Autodesk Inventor part; units mm, degrees
ref_plane "YZ Plane" through (0, 0, 0) normal (1, 0, 0) x (0, 1, 0)
ref_plane "XZ Plane" through (0, 0, 0) normal (0, 1, 0) x (-1, 0, 0)
ref_plane "XY Plane" through (0, 0, 0) normal (0, 0, 1) x (1, 0, 0)
sketch "Base" plane through (0, 0, 0) normal (0, 0, 1) x (1, 0, 0)
  circle A0 centre (0, 0) radius 25.4
  arc A1 (296.4611, -175.8738) -> (140.4514, -91.7589) centre (131.6761, -294.7694) ccw
  arc A2 (110.2711, -36.5273) -> (55.3611, 0.3584) centre (-26.1088, -180.2356) ccw
  arc A3 (110.2711, -36.5273) -> (151.7939, -57.2356) centre (164.9104, 21.0482) ccw
  arc A4 (244.1, -98.1325) -> (151.7939, -57.2356) centre (118.2154, -257.642) ccw
  arc A5 (244.1, -98.1325) -> (322.9398, -136.302) centre (369.9847, 61.3771) ccw
  arc A6 (339.7063, -172.5127) -> (322.9398, -136.302) centre (317.0592, -161.0119) ccw
  arc A7 (296.4611, -175.8738) -> (339.7063, -172.5127) centre (317.0592, -161.0119) ccw
  line L0 (128.6011, -96.3262) -> (140.4514, -91.7589)
  line L1 (0, 0) -> (317.0592, -161.0119) construction
  circle A8 centre (317.0592, -161.0119) radius 25.4 construction
  arc A9 (0, -25.4) -> (128.6011, -96.3262) centre (153.166, 100.265) ccw
  line L2 (0, 0) -> (0, -25.4) construction
  arc A10 (55.3611, 0.3584) -> (42.3326, -1.2004) centre (50.1387, -11.2181) ccw
  arc A11 (25.4, -0.0141) -> (42.3326, -1.2004) centre (34.5266, 8.8174) ccw
  line L3 (110.2711, -36.5273) -> (102.4101, -52.0068) construction
  line L4 (50.1387, -11.2181) -> (44.3883, -22.5417) construction
  line L5 (140.4514, -91.7589) -> (148.7008, -75.5146) construction
  line L6 (244.1, -98.1325) -> (233.6726, -118.6658) construction
  line L7 (339.7063, -172.5127) -> (317.0592, -161.0119) construction
  dimension "d101" = 50.8
  dimension "d98" = 355.6
  dimension "d99" = 203.2
  dimension "d100" = 79.375
  dimension "d102" = 198.12
  dimension "d103" = 50.8
  dimension "d104" = 12.7
  dimension "d105" = 203.2
  dimension "d106" = 48
  dimension "d107" = 12.7
  dimension "d108" = 12.7
  dimension "d109" = 23.495
  dimension "d111" = 158.75
  dimension "d112" = 222.25
  dimension "d113" = 49.784
  dimension "d114" = 65.0748
  dimension "d115" = 51.9176
  dimension "d116" = 95.3008
  dimension "d117" = 93.5228
extrude "Plate1" add sketch "Base" along normal blind 5
sketch "MountHoles" plane through (0, 0, 5) normal (0, 0, 1) x (1, 0, 0)
  arc A0 (296.4611, -175.8738) -> (322.9398, -136.302) centre (317.0592, -161.0119) ccw
  circle A1 centre (317.0592, -161.0119) radius 3.175
  circle A2 centre (0, 0) radius 3.175
  circle A3 centre (0, 0) radius 15.875 construction
  circle A4 centre (0, 15.875) radius 3.175
  line L0 (0, 15.875) -> (0, 0) construction
  circle A5 centre (-13.7482, 7.9375) radius 3.175
  circle A6 centre (-13.7482, -7.9375) radius 3.175
  circle A7 centre (0, -15.875) radius 3.175
  circle A8 centre (13.7482, -7.9375) radius 3.175
  circle A9 centre (13.7482, 7.9375) radius 3.175
  point P0 (278.6053, -195.7416)
  point P1 (14.9365, 6.9557)
  dimension "d40" = 31.75
  dimension "d38" = 6.35
  dimension "d39" = 6.35
  dimension "d43" = 360
hole "MountHolesFeature" at (0, 0, 5) direction (0, 0, -1) diameter 8 end through all
fillet "SmallFilletsFeature" radius 8 2 edges at (140.4514, -91.7589, 2.5) (128.6011, -96.3262, 2.5)
sketch "WheelMountHole" plane through (0, 0, 5) normal (0, 0, 1) x (1, 0, 0)
  arc A0 (296.4611, -175.8738) -> (322.9398, -136.302) centre (317.0592, -161.0119) ccw
  circle A1 centre (317.0592, -161.0119) radius 6.35
  point P0 (0, 0)
  point P1 (278.6053, -195.7416)
  dimension "d83" = 12.7
hole "WheelMountHoleFeature" at (317.0592, -161.0119, 5) direction (0, 0, -1) diameter 24.5 end through all
sketch "PistonMountHole" plane through (0, 0, 0) normal (0, 0, -1) x (-1, 0, 0)
  circle A0 centre (-195.6083, -86.6143) radius 3
  arc A1 (-151.7939, -57.2356) -> (-244.1, -98.1325) centre (-118.2154, -257.642) ccw
  line L0 (-206.4619, -74.6043) -> (-184.7548, -98.6243) construction
  arc A2 (-142.169, -91.8405) -> (-296.4611, -175.8738) centre (-131.6761, -294.7694) ccw
  point P0 (0, 0)
  dimension "d120" = 6
  dimension "d122" = 203.2
  dimension "d197" = 77.3929
extrude "PistonMountHoleFeature" cut sketch "PistonMountHole" against normal blind 5
sketch "MotorExtend" plane through (0, 0, 5) normal (0, 0, 1) x (1, 0, 0)
  circle A0 centre (70.2482, -45.9648) radius 36
  arc A1 (0, -25.4) -> (126.5447, -96.0583) centre (153.166, 100.265) ccw construction
  arc A2 (110.2711, -36.5273) -> (151.7939, -57.2356) centre (164.9104, 21.0482) ccw construction
  circle A3 centre (0, 0) radius 4
  line L0 (0, 0) -> (140.4963, -91.9296) construction
  arc A4 (142.169, -91.8405) -> (138.8789, -92.365) centre (141.7559, -99.8298) ccw
  arc A5 (0, -25.4) -> (46.966, -73.4228) centre (280.2614, 201.7164) ccw
  arc A6 (126.5447, -96.0583) -> (130.4966, -95.5956) centre (127.6196, -88.1308) ccw
  arc A7 (58.6335, -80.0397) -> (126.5447, -96.0583) centre (175.0163, 261.4034) ccw
  arc A8 (55.3611, 0.3584) -> (42.3326, -1.2004) centre (50.1387, -11.2181) ccw
  arc A9 (85.2601, -13.2441) -> (55.3611, 0.3584) centre (-2070.8473, -4712.7994) ccw
  arc A10 (110.2711, -36.5273) -> (55.3611, 0.3584) centre (-26.1088, -180.2356) ccw
  arc A11 (110.2711, -36.5273) -> (94.2542, -19.1374) centre (12.4591, -110.5454) ccw
  line L1 (0, -25.4) -> (55.3611, 0.3584)
  line L2 (110.2711, -36.5273) -> (126.5447, -96.0583)
  point P0 (70.2482, -45.9648)
  dimension "d128" = 72
sheet face with bend "MotorExtendFeature" sketch "MotorExtend" thickness 5 toward (0, 0, -1) bend radius 5 contours A0 A10 | A11 A10 A0 | A0 A10 A9 | A10 L2 A7 A0 | A0 A10 | A0 A5 L1 A10
bend "Bend1"
sketch "MotorCut" plane through (0, 0, 5) normal (0, 0, 1) x (1, 0, 0)
  circle A0 centre (70.2482, -45.9648) radius 36
  circle A1 centre (70.2482, -45.9648) radius 15
  point P0 (0, 0)
  dimension "d134" = 30
extrude "MotorCutFeature" cut sketch "MotorCut" against normal blind 5 contours A1
sketch "MotorMountHoles" plane through (0, 0, 5) normal (0, 0, 1) x (1, 0, 0)
  circle A0 centre (56.943, -61.9327) radius 3.5 construction
  circle A1 centre (63.0721, -26.4582) radius 3.5 construction
  circle A2 centre (90.7293, -49.5034) radius 3.5 construction
  circle A3 centre (63.0721, -26.4582) radius 2.5
  circle A4 centre (90.7293, -49.5034) radius 2.5
  circle A5 centre (56.943, -61.9327) radius 2.5
  point P0 (0, 0)
  dimension "d180" = 5
extrude "MotorMountHolesFeature" cut sketch "MotorMountHoles" against normal blind 5
sketch "HubCoverExtend" plane through (0, 0, 5) normal (0, 0, 1) x (1, 0, 0)
  circle A0 centre (317.0592, -161.0119) radius 12.25
  circle A1 centre (317.0592, -161.0119) radius 50.8
  arc A2 (244.1, -98.1325) -> (322.9398, -136.302) centre (369.9847, 61.3771) ccw
  arc A3 (296.4611, -175.8738) -> (142.169, -91.8405) centre (131.6761, -294.7694) ccw
  arc A4 (244.1, -98.1325) -> (305.2545, -111.6025) centre (288.573, -41.7804) ccw
  arc A5 (266.9914, -169.606) -> (228.8665, -116.3198) centre (192.9202, -182.3202) ccw
  point P0 (0, 0)
  point P1 (283.7795, -122.6308)
  point P2 (268.8853, -144.8899)
  dimension "d139" = 101.6
sheet face with bend "HubCoverExtendFeature" sketch "HubCoverExtend" thickness 5 toward (0, 0, -1) bend radius 5
bend "Bend2"
sketch "HubPressFitHole" plane through (0, 0, 5) normal (0, 0, 1) x (1, 0, 0)
  circle A0 centre (317.0592, -161.0119) radius 12.25
  circle A1 centre (317.0592, -161.0119) radius 35.9873
  point P0 (0, 0)
  dimension "d145" = 71.9746
extrude "HubPressFitHoleFeature" cut sketch "HubPressFitHole" against normal blind 5 contours A0 | A1
sketch "ShinThicken" plane through (0, 0, 5) normal (0, 0, 1) x (1, 0, 0)
  arc A0 (266.9914, -169.606) -> (228.8665, -116.3198) centre (192.9202, -182.3202) ccw
  arc A1 (228.8665, -116.3198) -> (142.169, -91.8405) centre (131.6761, -294.7694) ccw
  arc A2 (266.9914, -169.606) -> (142.169, -91.8405) centre (133.4629, -244.8745) ccw
  point P0 (0, 0)
sheet face with bend "ShinThickenFeature" sketch "ShinThicken" thickness 5 toward (0, 0, -1) bend radius 5
bend "Bend3"
fillet "BlendFilletFeature" radius 32 1 edges at (266.9914, -169.606, 2.5)
sketch "MotorMountExtension" plane through (0, 0, 5) normal (0, 0, 1) x (1, 0, 0)
  arc A0 (55.3611, 0.3584) -> (42.3326, -1.2004) centre (50.1387, -11.2181) ccw
  arc A1 (55.3611, 0.3584) -> (35.2473, 5.0627) centre (33.3341, -48.4687) ccw
  arc A2 (25.4, -0.0141) -> (0, -25.4) centre (0, 0) ccw
  arc A3 (21.8139, 13.0121) -> (35.2473, 5.0627) centre (35.8302, 21.3728) ccw
  arc A4 (85.2601, -13.2441) -> (55.3611, 0.3584) centre (-2070.8473, -4712.7994) ccw
  arc A5 (25.4, -0.0141) -> (42.3326, -1.2004) centre (34.5266, 8.8174) ccw
sheet face with bend "MotorMountExtensionFeature" sketch "MotorMountExtension" thickness 5 toward (0, 0, -1) bend radius 5
bend "Bend4"
sketch "HubMountHoles" plane through (0, 0, 0) normal (0, 0, -1) x (-1, 0, 0)
  circle A0 centre (3.7224, -11.408) radius 2 construction
  circle A1 centre (11.408, 3.7224) radius 2 construction
  circle A2 centre (-11.408, -3.7224) radius 2 construction
  circle A3 centre (-3.7224, 11.408) radius 2 construction
  circle A4 centre (-3.7224, 11.408) radius 1.7
  circle A5 centre (-11.408, -3.7224) radius 1.7
  circle A6 centre (3.7224, -11.408) radius 1.7
  circle A7 centre (11.408, 3.7224) radius 1.7
  point P0 (0, 0)
  dimension "d190" = 4
  dimension "d191" = 3.4
  dimension "d192" = 3.4
  dimension "d193" = 3.4
  dimension "d194" = 3.4
extrude "HubMountHolesFeature" cut sketch "HubMountHoles" against normal blind 5
sketch "EncoderMountHoles" plane through (0, 0, 0) normal (0, 0, -1) x (-1, 0, 0)
  circle A0 centre (-278.0337, -169.7877) radius 2.2
  circle A1 centre (-308.2834, -121.9864) radius 2.2
  circle A2 centre (-356.0846, -152.2361) radius 2.2
  circle A3 centre (-325.835, -200.0373) radius 2.2
  point P0 (0, 0)
extrude "EncoderMountHolesFeature" cut sketch "EncoderMountHoles" against normal blind 5
sketch "RollerGuideHole" plane through (0, 0, 5) normal (0, 0, 1) x (1, 0, 0)
  line L0 (99.8861, -66.3999) -> (106.0449, -83.3135) construction
  line L1 (102.705, -65.3734) -> (108.8638, -82.287)
  line L2 (103.2259, -84.3399) -> (97.0672, -67.4263)
  arc A0 (102.705, -65.3734) -> (97.0672, -67.4263) centre (99.8861, -66.3999) ccw
  arc A1 (103.2259, -84.3399) -> (108.8638, -82.287) centre (106.0449, -83.3135) ccw
  arc A2 (126.5447, -96.0583) -> (130.4966, -95.5956) centre (127.6196, -88.1308) ccw
  circle A3 centre (70.2482, -45.9648) radius 15
  circle A4 centre (0, 0) radius 4
  line L3 (0, 0) -> (70.2482, -45.9648) construction
  circle A5 centre (317.0592, -161.0119) radius 35.9873
  line L4 (317.0592, -161.0119) -> (70.2482, -45.9648) construction
  point P0 (102.9655, -74.8567)
  point P1 (128.5499, -96.0766)
  dimension "d200" = 3
  dimension "d205" = 18
  dimension "d206" = 45
  dimension "d207" = 6
  dimension "d208" = 36
extrude "RollerGuideHoleFeature" cut sketch "RollerGuideHole" against normal blind 5 contours L1 A1 L2 A0
equation "\"d66\" = Thickness"
equation "\"d89\" = Thickness"
equation "\"d37\" = Thickness"
equation "\"BendRadius\" = Thickness"
equation "\"BendReliefWidth\" = Thickness"
equation "\"BendReliefDepth\" = 0.5 * Thickness"
equation "\"TransitionRadius\" = BendRadius"
equation "\"JacobiRadiusSize\" = BendRadius"
equation "\"GapSize\" = Thickness"
properties part number "LowerLeg"
Could you check a few things on this model? Use its own coordinates, in mm. A direction names the side the tool comes from. Round coordinates to 2 decimals unless told otherwise and drop trailing zeros. Loops run counter-clockwise (first coordinate to the right, second up) from the corner with the lowest first, then second, coordinate; pieces in that order, holes last. Notation, with made-up numbers: (41.25, -5) -> (90.25, -5) arc R18 cw to (90.25, 1) -> close; hole circle Ø7 at (52, 28.5). An arc over 180 degrees is marked (long way). Put each result on its own line as item: value.
Q1. I want a section at C-C on x = 223. Write out the boundary of the cut face in (y, z).
Checks:
outline: (-120.46, 0) -> (-83.54, 0) -> (-83.54, 5) -> (-120.46, 5) -> close
Q2. Please list where these lines run through material, in increasing order: line 1 (Y direction, x = 326.5, z = 3.85) (3 decimals); line 2 (X direction, y = -153.5, z = 3.3); line 3 (Y direction, x = 10, z = 3.25). Write a range as from..to.
Checks:
line 1: -210.927..-202.134, -197.94..-195.739, -126.285..-111.097
line 2: 256.53..281.86, 352.25..354.28, 357.89..367.3
line 3: -37.21..-4.68, -2.77..23.35
Q3. I want a section at D-D on y = -104. Write out the boundary of the cut face in (x, z).
Checks:
outline: (193.87, 0) -> (252.77, 0) -> (252.77, 5) -> (193.87, 5) -> close
Q4. Which directions (+Z, -Z, +X, -X, +Y, -Y) give clear straight access to the entire face, cutting with the end or side of a thin tool? Please do faces 4 (the cylindrical face through (27.4, 7.4, 2.5)), 5 (the cylindrical face through (212.949, -113.813, 2.535)).
Checks:
face 4: +Z, -Z, +X, +Y
face 5: +Z, -Z, -Y
Q5. For pin 1 Ø3.5 at (x, y) = (325.83, -200.04) entering from -Z; pin 2 Ø1 at (y, z) = (-184.5, 2.5) entering from -X; pin 3 Ø1 at (y, z) = (-18.5, 1) entering from -X; pin 4 Ø3 at (x, z) = (172, 2) entering from -Y, each with a flat end and sliding along its axis, tell me the tip position at first contact or that it passes through.
Checks:
pin 1: through
pin 2: x = 271.76
pin 3: x = -17.92
pin 4: y = -96.91
Q6. Thinking about a two-plate mould opening in Y: for faces 1 (the flat face through (156, -84, 0)), 2 (the cylindrical face through (3.905, 0.867, 2.465)), 3 (the cylindrical face through (22.034, -50.17, 2.535)), which applies, pulls with the +Y half, pulls with the -Y half, needs draft (parallel to the pull), parting line crosses it, or undercut?
Checks:
face 1: needs draft
face 2: undercut
face 3: pulls with the -Y half
Q7. I want a section at A-A on x = 296. Write out the boundary of the cut face in (y, z), and give its area (3 significant figures).
Checks:
outline: (-207.24, 0) -> (-190.19, 0) -> (-190.19, 5) -> (-207.24, 5) -> close; (-131.83, 0) -> (-113.18, 0) -> (-113.18, 5) -> (-131.83, 5) -> close
area: 178 mm2
Q8. I want a section at B-B on z = 2.4. Give the number of separate pieces and of enclosed holes in the cut face, and give its area (3 significant figures).
Checks:
separate pieces: 1
enclosed holes: 16
area: 18,300 mm2
